```python
from build123d import *

# Parameters (mm, degrees)
SKETCH2_R           = 0.4
BOSS_EXTRUDE1_DEPTH = 0.2


with BuildPart() as part:
    # Sketch2 → Boss-Extrude1 (new body)
    with BuildSketch(Plane(origin=(0, 0, 0), x_dir=(1, 0, 0), z_dir=(0, 1, 0))):
        with BuildLine():
            ThreePointArc((2.988962385, -3.562106661), (0, 4.65), (-2.988962385, -3.562106661))
            ThreePointArc((-2.988962385, -3.562106661), (-1.721013538, -3.45117551), (-1.831944688, -2.183226663))
            ThreePointArc((-1.831944688, -2.183226663), (0, 2.85), (1.831944688, -2.183226663))
            ThreePointArc((1.831944688, -2.183226663), (1.721013538, -3.45117551), (2.988962385, -3.562106661))
        make_face()
        with Locations(Location((-2.410453536, -2.872666662, 0), (0, 0, 270))):
            Circle(SKETCH2_R, mode=Mode.SUBTRACT)
        with Locations(Location((2.410453536, -2.872666662, 0), (0, 0, 270))):
            Circle(SKETCH2_R, mode=Mode.SUBTRACT)
    extrude(amount=BOSS_EXTRUDE1_DEPTH)


solid = part.part
```
Could you check a few things on this model? Use its own coordinates, in mm. Round coordinates to 2 decimals unless told otherwise and drop trailing zeros. Loops run counter-clockwise (first coordinate to the right, second up) from the corner with the lowest first, then second, coordinate; pieces in that order, holes last. Notation, with made-up numbers: (-5, 68) - (7, 68) arc R28 ccw to (7, 91) - close; hole circle Ø3 at (54.5, 52.25). An arc over 180 degrees is marked (long way). Answer as CSV lines item,"result".
1. Please list where these lines run through material, in increasing order: line 1 along Z through (x, y) = (2.5, 0.15); line 2 along X through (y, z) = (0.1, 0); line 3 along X through (y, z) = (0.1, 2). Write a range as [from, to].
Filled in:
line 1,"z = [-3.92, -1.37], [1.37, 2.48], [3.26, 3.77]"
line 2,"x = [-4.65, -2.85], [2.85, 4.65]"
line 3,"x = [-4.2, -2.03], [2.03, 4.2]"
2. I want a section at D-D on x = 0. List the corners of the cut face in (y, z) for me.
Filled in:
outline,"(0, -4.65) - (0.2, -4.65) - (0.2, -2.85) - (0, -2.85) - close"
3. I want a section at A-A on z = 0. List the corners of the cut face in (x, y) for me, then the cut area to 3 significant figures.
Filled in:
outline,"(-4.65, 0) - (-2.85, 0) - (-2.85, 0.2) - (-4.65, 0.2) - close; (2.85, 0) - (4.65, 0) - (4.65, 0.2) - (2.85, 0.2) - close"
area,"0.720 mm^2"
4. For pin 1 Ø3 at (x, z) = (0, -0.5) entering from -Y, with a flat end and sliding along its axis, tell me the tip position at first contact or that it passes through.
Filled in:
pin 1,"passes through"
5. I want a section at B-B on y = 0.05. List the corners of the cut face in (x, z) for me, then the cut area to 3 significant figures.
Filled in:
outline,"(-2.99, 3.56) arc R4.65 ccw (long way) to (2.99, 3.56) arc R0.9 ccw to (1.83, 2.18) arc R2.85 cw (long way) to (-1.83, 2.18) arc R0.9 ccw to start; hole circle Ø0.8 at (-2.41, 2.87); hole circle Ø0.8 at (2.41, 2.87)"
area,"34.5 mm^2"
6. I want a section at C-C on z = -2. List the corners of the cut face in (x, y) for me, then the cut area to 3 significant figures.
Filled in:
outline,"(-4.2, 0) - (-2.03, 0) - (-2.03, 0.2) - (-4.2, 0.2) - close; (2.03, 0) - (4.2, 0) - (4.2, 0.2) - (2.03, 0.2) - close"
area,"0.867 mm^2"
